Could you check a few things on this model? Use its own coordinates, in mm. A direction names the side the tool comes from. Give positions to 0.01 mm unless a question says otherwise; leave off trailing zeros. Write each loop counter-clockwise with the first axis right and the second up, starting at its lowest first coordinate (ties: lowest second). Pieces come first, ordered by that corner, then holes. Notation, with made-up numbers: (72, 48.5) - (80, 48.5) arc R27 cw to (80, 67.5) - close; hole circle Ø3 at (54, 69). An arc over 180 degrees is marked (long way). Use one line per item in the form item = value.
```python
from build123d import *

# Parameters (mm, degrees)
SKETCH1_R           = 1.05
BOSS_EXTRUDE1_DEPTH = 3
SKETCH2_W           = 4
SKETCH2_H           = 8.44
BOSS_EXTRUDE2_DEPTH = 10
SKETCH3_R           = 1.3
CUT_EXTRUDE1_DEPTH  = 57.893656061
FILLET1_R           = 3
FILLET6_R           = 1.5


with BuildPart() as part:
    # Sketch1 → Boss-Extrude1 (new body)
    with BuildSketch(Plane(origin=(0, 0, 0), x_dir=(1, 0, 0), z_dir=(0, 1, 0))):
        with BuildLine():
            Line((0, 0), (24.457992021, 0))
            ThreePointArc((24.457992021, 0), (25.872205583, 0.585786438), (26.457992021, 2))
            Line((26.457992021, 2), (26.457992021, 14))
            Line((26.457992021, 14), (22.081671712, 14))
            ThreePointArc((22.081671712, 14), (21.102023762, 13.743642708), (20.373515707, 13.040289893))
            Line((20.373515707, 13.040289893), (16.542468334, 6.749710107))
            ThreePointArc((16.542468334, 6.749710107), (15.813960279, 6.046357292), (14.834312329, 5.79))
            Line((14.834312329, 5.79), (-15.508328288, 5.79))
            ThreePointArc((-15.508328288, 5.79), (-16.487976238, 6.046357292), (-17.216484293, 6.749710107))
            Line((-17.216484293, 6.749710107), (-21.047531666, 13.040289893))
            ThreePointArc((-21.047531666, 13.040289893), (-21.776039721, 13.743642708), (-22.755687671, 14))
            Line((-22.755687671, 14), (-27.132007979, 14))
            Line((-27.132007979, 14), (-27.132007979, 2))
            ThreePointArc((-27.132007979, 2), (-26.546221542, 0.585786438), (-25.132007979, 0))
            Line((-25.132007979, 0), (0, 0))
        make_face()
        with Locations(Location((18.957992021, 3.23, 0), (0, 0, 270))):
            Circle(SKETCH1_R, mode=Mode.SUBTRACT)
        with Locations(Location((-19.632007979, 3.23, 0), (0, 0, 270))):
            Circle(SKETCH1_R, mode=Mode.SUBTRACT)
    extrude(amount=BOSS_EXTRUDE1_DEPTH)

    # Sketch2 → Boss-Extrude2 (add)
    with BuildSketch(Plane(origin=(0, 3, 0), x_dir=(1, 0, 0), z_dir=(0, 1, 0))):
        with Locations((-25.132007979, 9.78)):
            Rectangle(SKETCH2_W, SKETCH2_H)
        with Locations((24.457992021, 9.78)):
            Rectangle(SKETCH2_W, SKETCH2_H)
    extrude(amount=BOSS_EXTRUDE2_DEPTH)

    # Sketch3 → Cut-Extrude1 (cut, through all)
    with BuildSketch(Plane(origin=(26.457992021, 0, 0), x_dir=(0, 0, -1), z_dir=(1, 0, 0))):
        with BuildLine():
            Line((10.68, 13), (8.88, 13))
            Line((8.88, 13), (8.88, 8.938083152))
            ThreePointArc((8.88, 8.938083152), (9.78, 9.3), (10.68, 8.938083152))
            Line((10.68, 8.938083152), (10.68, 13))
        make_face()
        with Locations((9.78, 8)):
            Circle(SKETCH3_R)
    extrude(amount=-CUT_EXTRUDE1_DEPTH, mode=Mode.SUBTRACT)

    # Fillet1
    fillet1_edges = [part.edges().sort_by_distance(p)[0] for p in [
        (-25.132007979, 8.938083152, -10.68),
        (24.457992021, 8.938083152, -10.68),
        (-25.132007979, 8.938083152, -8.88),
        (24.457992021, 8.938083152, -8.88),
    ]]
    fillet(fillet1_edges, radius=FILLET1_R)

    # Fillet6
    fillet6_edges = [part.edges().sort_by_distance(p)[0] for p in [
        (-25.132007979, 13, -5.56),
        (-25.132007979, 13, -14),
        (24.457992021, 13, -14),
        (24.457992021, 13, -5.56),
        (24.457992021, 13, -10.68),
        (24.457992021, 13, -8.88),
        (-25.132007979, 13, -8.88),
        (-25.132007979, 13, -10.68),
    ]]
    fillet(fillet6_edges, radius=FILLET6_R)


solid = part.part
```
1. Which directions (+Z, -Z, +X, -X, +Y, -Y) give clear straight access to the entire face, cutting with the end or side of a thin tool? Please do faces 1 (the face through (-23.132, 6.8, -8.8)), 2 (the face through (24, 11, -10.68)), 3 (the face through (0, 1, -5.79)).
Response values:
face_1 = +Z, -Z, +Y
face_2 = +X, -X, +Y
face_3 = -Z, +Y, -Y
2. If we mould it in two halves opening along Y, with no side actions, what happens to faces 4 (the face through (24.49, 12.55, -13.57)), 5 (the face through (24.43, 9.16, -8.81)), 6 (the face through (21.11, 1.48, -13.75))? For each: pulls with the +Y half, pulls with the -Y half, needs draft (parallel to the pull), parting line crosses it, or undercut.
Response values:
face_4 = pulls with the +Y half
face_5 = undercut
face_6 = needs draft
3. For pin 1 (2 mm diameter, centred on x = -25, y = 6, fed in from +Z); pin 2 (6 mm diameter, centred on x = -16, y = 4.5, fed in from -Z); pin 3 (1.5 mm diameter, centred on x = -4.5, y = 2, fed in from -Z), each with a flat end and sliding along its axis, tell me the tip position at first contact or that it passes through.
Response values:
pin_1 = -5.56
pin_2 = -9.02
pin_3 = -5.79
4. Imagine slicing it at C-C, the plane z = -9.5. List the corners of the cut face in (x, y) for me.
Response values:
outline = (-27.13, 0) - (-18.89, 0) - (-18.89, 3) - (-23.13, 3) - (-23.13, 6.73) - (-27.13, 6.73) - close; (18.22, 0) - (26.46, 0) - (26.46, 6.73) - (22.46, 6.73) - (22.46, 3) - (18.22, 3) - close
5. Imagine slicing it at B-B, the plane z = -3.23. List the corners of the cut face in (x, y) for me, and give its area (3 significant figures).
Response values:
outline = (-27.13, 0) - (-20.68, 0) - (-20.68, 3) - (-27.13, 3) - close; (-18.58, 0) - (17.91, 0) - (17.91, 3) - (-18.58, 3) - close; (20.01, 0) - (26.46, 0) - (26.46, 3) - (20.01, 3) - close
area = 148 mm²
6. If I drill on line 1 (X direction, y = 9.75, z = -12.75); line 2 (Z direction, x = 24.75, y = 8); line 3 (Z direction, x = -13, y = 0.5), over which ranges is the centre line in solid material (lowest first)? Write a range as from..to.
Response values:
line_1 = -27.13..-23.13, 22.46..26.46
line_2 = -14..-11.08, -8.48..-5.56
line_3 = -5.79..0
7. Imagine slicing it at A-A, the plane y = 8. List the corners of the cut face in (x, z) for me, and give its area (3 significant figures).
Response values:
outline = (-27.13, -14) - (-23.13, -14) - (-23.13, -11.08) - (-27.13, -11.08) - close; (-27.13, -8.48) - (-23.13, -8.48) - (-23.13, -5.56) - (-27.13, -5.56) - close; (22.46, -14) - (26.46, -14) - (26.46, -11.08) - (22.46, -11.08) - close; (22.46, -8.48) - (26.46, -8.48) - (26.46, -5.56) - (22.46, -5.56) - close
area = 46.7 mm²
8. Imagine slicing it at D-D, the plane x = -10. List the corners of the cut face in (y, z) for me, and give its area (3 significant figures).
Response values:
outline = (0, -5.79) - (3, -5.79) - (3, 0) - (0, 0) - close
area = 17.4 mm²
